Check sheet for the modelled part. Datum: model origin and axes. Units: mm. A direction names the side the tool comes from. Round coordinates to 2 decimals unless told otherwise and drop trailing zeros. Order: outer loops, then holes, each group sorted by start corner. A loop starts at its lowest first (then second) coordinate and runs counter-clockwise, first axis right, second up.
```python
from build123d import *

# Parameters (mm, degrees)
CHAMFER_1_SIZE = 1


with BuildPart() as part:
    # 草图1 → 旋转1 (revolve)
    with BuildSketch(Plane.XY):
        Polygon((0, 10.5), (0, 0), (82, 0), (82, 8), (77.2, 8), (77.2, 7.35), (76.2, 7.35), (76.2, 8), (8, 8), (8, 6.691876128), (6, 6.691876128), (6, 8), (6, 10.5), align=None)
    revolve(axis=Axis((82, 0, 0), (-1, 0, 0)))

    # 倒角1
    chamfer_1_edges = [part.edges().sort_by_distance(p)[0] for p in [
        (82, -8, 0),
        (0, -10.5, 0),
    ]]
    chamfer(chamfer_1_edges, length=CHAMFER_1_SIZE)


solid = part.part
```
Item 1: Sectioned sample at C-C (x = 66). Record the cut outline in (y, z).
Answer:
outline: circle Ø16 at (0, 0)
Item 2: Scan lines: line 1 along X through (y, z) = (4.5, 5.25); line 2 along X through (y, z) = (-4.5, 6.5); line 3 along X through (y, z) = (4, 8.25). Record each from-to range of solid material in increasing order.
Answer:
line 1: x = 0 to 6, 8 to 82
line 2: x = 0 to 6, 8 to 76.2, 77.2 to 81.09
line 3: x = 0 to 6
Item 3: Access from +Z, -Z, +X, -X, +Y, -Y to the whole of each face (thin tool, end or side, straight path). Record for faces 1 (the cylindrical face through (6.986, 6.383, -2.01)), 2 (the flat face through (0, 0, 0)), 3 (the cylindrical face through (79.07, -1.73, 7.81)).
Answer:
face 1: none
face 2: +Z, -Z, -X, +Y, -Y
face 3: +X
Item 4: Go/stop test with flat-tipped pins: P1, Ø3, axis at x = 34.5, y = -8, coming from the -Z side; P2, Ø4, axis at x = 27, y = -8, coming from the -Z side; P3, Ø5, axis at x = 42, y = -8.5, coming from the +Z side; P4, Ø4, axis at y = 1.5, z = -5.5, coming from the -X side. Record where each tip stops, or that it passes through.
Answer:
P1: stops at z = -4.66
P2: stops at z = -5.29
P3: stops at z = 5.29
P4: stops at x = 0
Item 5: Sectioned sample at A-A (y = 0). Record the cut outline in (x, z).
Answer:
outline: (0, -9.5) - (1, -10.5) - (6, -10.5) - (6, -6.69) - (8, -6.69) - (8, -8) - (76.2, -8) - (76.2, -7.35) - (77.2, -7.35) - (77.2, -8) - (81, -8) - (82, -7) - (82, 7) - (81, 8) - (77.2, 8) - (77.2, 7.35) - (76.2, 7.35) - (76.2, 8) - (8, 8) - (8, 6.69) - (6, 6.69) - (6, 10.5) - (1, 10.5) - (0, 9.5) - close
Item 6: Release check for a two-part mould opening along X. For faces 4 (the cylindrical face through (3.5, 10, -3.2)), 5 (the flat face through (82, 0, 0)), 6 (the flat face through (8, -5, 5)) record: released by +X, released by -X, zero draft, split by the parting line, or undercut.
Answer:
face 4: zero draft
face 5: released by +X
face 6: undercut
